```python
from build123d import *

# Parameters (mm, degrees)
SKETCH1_W   = 1
SKETCH1_H   = 3.454401077
SKETCH1_W_2 = 1.75
SKETCH1_H_2 = 0.97


with BuildPart() as part:
    # Sketch1 → Revolve1 (revolve)
    with BuildSketch(Plane.XY, mode=Mode.PRIVATE) as revolve1_sk:
        Polygon((0, 0), (0, 1.145), (4, 3.454401077), (4, 0), align=None)
        with Locations((4.5, 1.727200539)):
            Rectangle(SKETCH1_W, SKETCH1_H)
        with Locations((5.875, 0.485)):
            Rectangle(SKETCH1_W_2, SKETCH1_H_2)
    revolve1 = revolve(revolve1_sk.sketch.rotate(Axis((0, 0, 0), (1, 0, 0)), 90), axis=Axis((0, 0, 0), (1, 0, 0)))

    # Mirror1: Revolve1 across plane
    add(revolve1.mirror(Plane(origin=(0, 0, 0), x_dir=(0, 0, 1), z_dir=(1, 0, 0))))


solid = part.part
```
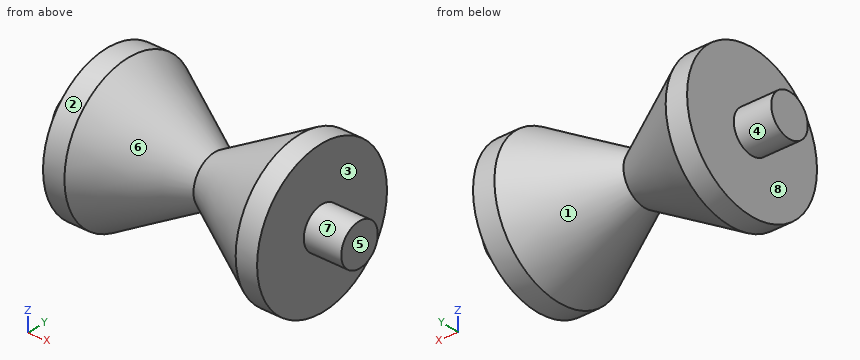
Geometry: final body of the model. Coordinates: model frame, mm. Face numbers are marked on the shaded views. A direction names the side the tool comes from. Coordinates: 2 decimals unless noted, no trailing zeros. Loops run counter-clockwise (first coordinate to the right, second up) from the corner with the lowest first, then second, coordinate; pieces in that order, holes last. Notation, with made-up numbers: (65, 68.5) -> (93, 68.5) arc R28 ccw to (93, 96.5) -> close; hole circle Ø10 at (68, 77.5). An arc over 180 degrees is marked (long way). Use a Markdown table: item, result. Add a question column.
(1) Section query A-A, the plane y = 0. Return loops of the section in (x, z) (3 decimals), plus the area to 3 significant figures.
(2) Section query C-C, the plane x = 4.25. Return loops of the section in (y, z), plus the area to 3 significant figures.
(3) Pin query (flat end, axial travel): pin 1 Ø2 at (y, z) = (0, -2.5) entering from -X; pin 2 Ø2 at (x, y) = (2.5, 1) entering from +Z; pin 3 Ø1.5 at (x, y) = (1.5, 1.5) entering from -Z. Return the tip coordinate at first contact, or that it passes through.
(4) Section query D-D, the plane x = 0.75. Return loops of the section in (y, z).
(5) Access query for the marked faces 1, 2, 3, 4 and 5. Directions: +Z, -Z, +X, -X, +Y, -Y. A direction counts if a zero-diameter tool reaches every point of the face in a straight line with its end or side. Return the directions, or none.
(6) Line query: line 1 along X through (y, z) = (1, -3); line 2 along X through (y, z) = (1.5, 0); line 3 along Y through (x, z) = (2.25, -1.5). Output: solid intervals per line, ascending.
(7) Mould query, pull axis X, two halves, no side actions, for the marked faces 6, 7 and 8. Classes: pulls with the +X half, pulls with the -X half, needs draft (parallel to the pull), parting line crosses it, or undercut.
Answer:
| question | item | result |
|---|---|---|
| 1 | outline | (-6.75, -0.97) -> (-5, -0.97) -> (-5, -3.454) -> (-4, -3.454) -> (0, -1.145) -> (4, -3.454) -> (5, -3.454) -> (5, -0.97) -> (6.75, -0.97) -> (6.75, 0.97) -> (5, 0.97) -> (5, 3.454) -> (4, 3.454) -> (0, 1.145) -> (-4, 3.454) -> (-5, 3.454) -> (-5, 0.97) -> (-6.75, 0.97) -> close |
| 1 | area | 57.4 mm^2 |
| 2 | outline | circle Ø6.91 at (0, 0) |
| 2 | area | 37.5 mm^2 |
| 3 | pin 1 | stops at x = -5 |
| 3 | pin 2 | stops at z = 3.06 |
| 3 | pin 3 | stops at z = -2.11 |
| 4 | outline | circle Ø3.16 at (0, 0) |
| 5 | face 1 | none |
| 5 | face 2 | +X, -X |
| 5 | face 3 | +X |
| 5 | face 4 | -X |
| 5 | face 5 | +Z, -Z, +X, +Y, -Y |
| 6 | line 1 | x = -5 to -3.49, 3.49 to 5 |
| 6 | line 2 | x = -5 to -0.61, 0.61 to 5 |
| 6 | line 3 | y = -1.93 to 1.93 |
| 7 | face 6 | undercut |
| 7 | face 7 | needs draft |
| 7 | face 8 | pulls with the -X half |
